Can you work these out from the drawing? Everything is in mm from the part's minimum corner. A direction names the side the tool comes from. Coordinates: 2 decimals unless noted, no trailing zeros. Loops run counter-clockwise (first coordinate to the right, second up) from the corner with the lowest first, then second, coordinate; pieces in that order, holes last.
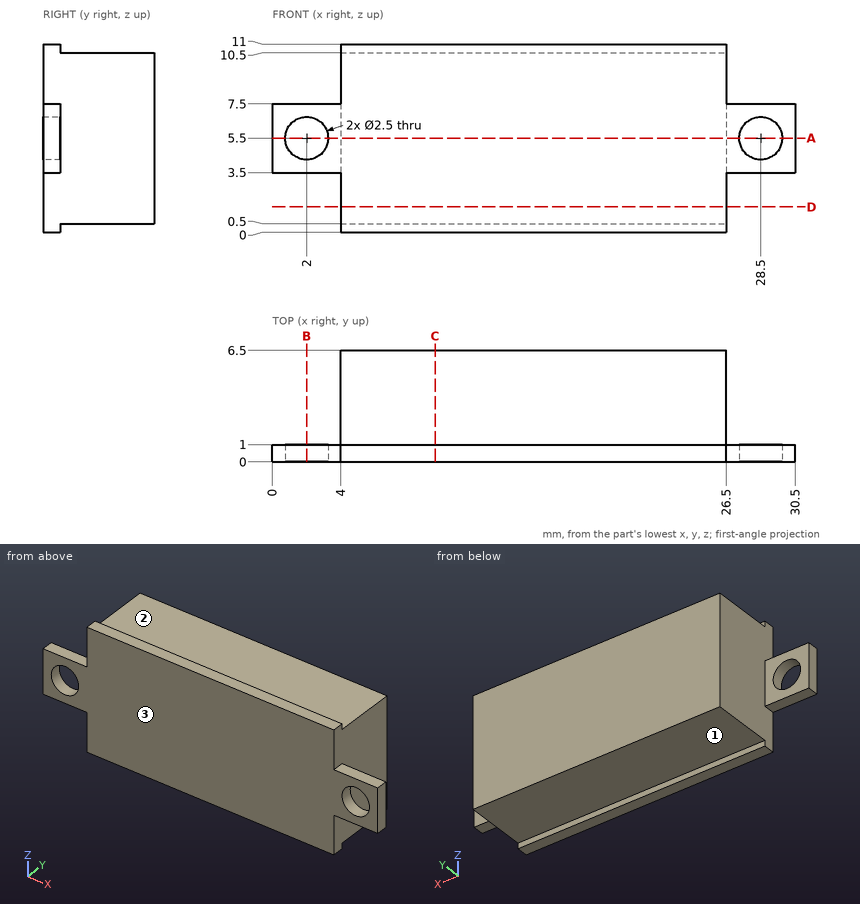
(1) Imagine slicing it at C-C, the plane x = 9.5. Write out the boundary of the cut face in (y, z), and give its area (3 significant figures).
Answers:
outline: (0, 0) - (1, 0) - (1, 0.5) - (6.5, 0.5) - (6.5, 10.5) - (1, 10.5) - (1, 11) - (0, 11) - close
area: 66.0 mm2
(2) Imagine slicing it at B-B, the plane x = 2. Write out the boundary of the cut face in (y, z).
Answers:
outline: (0, 3.5) - (1, 3.5) - (1, 4.25) - (0, 4.25) - close; (0, 6.75) - (1, 6.75) - (1, 7.5) - (0, 7.5) - close
(3) Imagine slicing it at A-A, the plane z = 5.5. Write out the boundary of the cut face in (x, y).
Answers:
outline: (0, 0) - (0.75, 0) - (0.75, 1) - (0, 1) - close; (3.25, 0) - (27.25, 0) - (27.25, 1) - (26.5, 1) - (26.5, 6.5) - (4, 6.5) - (4, 1) - (3.25, 1) - close; (29.75, 0) - (30.5, 0) - (30.5, 1) - (29.75, 1) - close
(4) Imagine slicing it at D-D, the plane z = 1.5. Write out the boundary of the cut face in (x, y).
Answers:
outline: (4, 0) - (26.5, 0) - (26.5, 6.5) - (4, 6.5) - close
(5) Which directions (+Z, -Z, +X, -X, +Y, -Y) give clear straight access to the entire face, cutting with the end or side of a thin tool? Please do the marked faces 1, 2 and 3.
Answers:
face 1: -Z, +X, -X, +Y
face 2: +Z, +X, -X, +Y
face 3: +Z, -Z, +X, -X, -Y
(6) For pin 1 (1.5 mm diameter, centred on x = 13, y = 5.5, fed in from -Z); pin 2 (1 mm diameter, centred on x = 9.5, y = 5, fed in from +Z); pin 3 (1.5 mm diameter, centred on x = 28.5, z = 5.5, fed in from +Y); pin 4 (2 mm diameter, centred on y = 3, z = 7, fed in from -X), each with a flat end and sliding along its axis, tell me the tip position at first contact or that it passes through.
Answers:
pin 1: stops at z = 0.5
pin 2: stops at z = 10.5
pin 3: passes through
pin 4: stops at x = 4
(7) I need wall thicknesses on probe 1 along X at (y, z) = (0.8, 5.5); probe 2 along X at (y, z) = (4.5, 4); probe 3 along Z at (x, y) = (14, 3). Which ranges of each line are inside material? Lowest first, please.
Answers:
probe 1: x = 0 to 0.75, 3.25 to 27.25, 29.75 to 30.5
probe 2: x = 4 to 26.5
probe 3: z = 0.5 to 10.5
